```python
from build123d import *

# Parameters (mm, degrees)
F0_R     = 1.5
F1_DEPTH = 2


with BuildPart() as f1:
    # F0 (on Top) → F1 (new body)
    with BuildSketch(Plane.XY):
        with BuildLine():
            Line((65, 3.5), (65, 37))
            ThreePointArc((65, 37), (61.5, 40.5), (58, 37))
            Line((58, 37), (58, 3.5))
            Line((58, 3.5), (0, 3.5))
            ThreePointArc((0, 3.5), (-3.5, 0), (0, -3.5))
            Line((0, -3.5), (71.5, -3.5))
            ThreePointArc((71.5, -3.5), (75, 0), (71.5, 3.5))
            Line((71.5, 3.5), (65, 3.5))
        make_face()
        Circle(F0_R, mode=Mode.SUBTRACT)
        with Locations((71.5, 0)):
            Circle(F0_R, mode=Mode.SUBTRACT)
        with Locations((61.5, 37)):
            Circle(F0_R, mode=Mode.SUBTRACT)
    extrude(amount=F1_DEPTH)


solid = f1.part
```
Geometry: final body of the model. Coordinates: model frame, mm. A direction names the side the tool comes from. Round coordinates to 2 decimals unless told otherwise and drop trailing zeros. Order: outer loops, then holes, each group sorted by start corner. A loop starts at its lowest first (then second) coordinate and runs counter-clockwise, first axis right, second up. Notation, with made-up numbers: (-13, 1.25) -> (22, 1.25) arc R8 ccw to (22, 15.25) -> close; hole circle Ø10 at (-26.5, -30.5). An arc over 180 degrees is marked (long way). Write each question's results on one line, items separated by ' | '.
Q1. Ray query, line 1 along Y through (x, z) = (71.5, 1.05); line 2 along Y through (x, z) = (61.5, 1.05); line 3 along X through (y, z) = (27, 0.4). Return the intervals inside material, ascending.
Response values:
line 1: -3.5 to -1.5, 1.5 to 3.5 | line 2: -3.5 to 35.5, 38.5 to 40.5 | line 3: 58 to 65
Q2. Section query C-C (z = 0.7). Output: boundary loops of the cut face in (x, y).
Response values:
outline: (0, -3.5) -> (71.5, -3.5) arc R3.5 ccw to (71.5, 3.5) -> (65, 3.5) -> (65, 37) arc R3.5 ccw to (58, 37) -> (58, 3.5) -> (0, 3.5) arc R3.5 ccw to start; hole circle Ø3 at (0, 0); hole circle Ø3 at (61.5, 37); hole circle Ø3 at (71.5, 0)
Q3. Section query D-D (x = 33). Output: boundary loops of the cut face in (y, z).
Response values:
outline: (-3.5, 0) -> (3.5, 0) -> (3.5, 2) -> (-3.5, 2) -> close
Q4. Pull-direction query (Y, two-part tool) for faces 1 (the face through (68, 3.5, 1)), 2 (the face through (65, 20, 1)), 3 (the face through (73, 0, 1)); classes: released by +Y, released by -Y, zero draft, split by the parting line, or undercut.
Response values:
face 1: released by +Y | face 2: zero draft | face 3: undercut
Q5. Pin query (flat end, axial travel): pin 1 Ø1 at (y, z) = (6, 1) entering from +X; pin 2 Ø0.6 at (x, z) = (26.5, 1) entering from +Y. Return the tip coordinate at first contact, or that it passes through.
Response values:
pin 1: x = 65 | pin 2: y = 3.5
Q6. Access query for faces 4 (the face through (-3.5, 0.1, 1)), 5 (the face through (29, 3.5, 1)). Directions: +Z, -Z, +X, -X, +Y, -Y. A direction counts if a zero-diameter tool reaches every point of the face in a straight line with its end or side. Return the directions, or none.
Response values:
face 4: +Z, -Z, -X | face 5: +Z, -Z, -X, +Y
Q7. Section query A-A (y = 0). Output: boundary loops of the cut face in (x, z).
Response values:
outline: (-3.5, 0) -> (-1.5, 0) -> (-1.5, 2) -> (-3.5, 2) -> close; (1.5, 0) -> (70, 0) -> (70, 2) -> (1.5, 2) -> close; (73, 0) -> (75, 0) -> (75, 2) -> (73, 2) -> close
Q8. Section query B-B (x = 61.5). Output: boundary loops of the cut face in (y, z), and give its area (3 significant figures).
Response values:
outline: (-3.5, 0) -> (35.5, 0) -> (35.5, 2) -> (-3.5, 2) -> close; (38.5, 0) -> (40.5, 0) -> (40.5, 2) -> (38.5, 2) -> close | area: 82.0 mm²
